```python
from build123d import *

# Parameters (mm, degrees)
BOSS_EXTRUDE1_DEPTH = 10
SKETCH3_R           = 2.25
SKETCH3_R_2         = 3
CUT_EXTRUDE1_DEPTH  = 10
SKETCH5_R           = 4
CUT_EXTRUDE2_DEPTH  = 5


with BuildPart() as part:
    # Sketch2 → Boss-Extrude1 (new body)
    with BuildSketch(Plane(origin=(0, 0, 0), x_dir=(1, 0, 0), z_dir=(0, 1, 0))):
        Polygon((0, -34), (34, 0), (94, 0), (94, -94), (0, -94), align=None)
    extrude(amount=BOSS_EXTRUDE1_DEPTH)

    # Sketch3 → Cut-Extrude1 (cut)
    with BuildSketch(Plane(origin=(0, 10, 0), x_dir=(1, 0, 0), z_dir=(0, 1, 0))):
        with Locations((58.75, -6.25)):
            Circle(SKETCH3_R)
        with Locations((87.75, -35.25)):
            Circle(SKETCH3_R)
        with Locations((6.25, -62.75)):
            Circle(SKETCH3_R)
        with Locations((31.25, -87.75)):
            Circle(SKETCH3_R)
        with Locations((6, -88)):
            Circle(SKETCH3_R_2)
        with BuildLine():
            Line((90.828427125, -7.414213562), (89.414213562, -8.828427125))
            ThreePointArc((89.414213562, -8.828427125), (85.171572875, -8.828427125), (85.171572875, -4.585786438))
            Line((85.171572875, -4.585786438), (86.585786438, -3.171572875))
            ThreePointArc((86.585786438, -3.171572875), (90.828427125, -3.171572875), (90.828427125, -7.414213562))
        make_face()
    extrude(amount=-CUT_EXTRUDE1_DEPTH, mode=Mode.SUBTRACT)

    # Sketch5 → Cut-Extrude2 (cut)
    with BuildSketch(Plane(origin=(0, 10, 0), x_dir=(1, 0, 0), z_dir=(0, 1, 0))):
        with Locations((58.75, -6.25)):
            Circle(SKETCH5_R)
        with Locations((87.75, -35.25)):
            Circle(SKETCH5_R)
        with Locations((6.25, -62.75)):
            Circle(SKETCH5_R)
        with Locations((31.25, -87.75)):
            Circle(SKETCH5_R)
    extrude(amount=-CUT_EXTRUDE2_DEPTH, mode=Mode.SUBTRACT)


solid = part.part
```
Model file for the job. Use its own axes, mm. A direction names the side the tool comes from. Coordinates: 2 decimals unless noted, no trailing zeros. Order: outer loops, then holes, each group sorted by start corner. A loop starts at its lowest first (then second) coordinate and runs counter-clockwise, first axis right, second up. Notation, with made-up numbers: (48, -5.5) -> (87, -5.5) arc R26 cw to (87, 10.5) -> close; hole circle Ø5 at (-28.75, -10.75). An arc over 180 degrees is marked (long way). Answer as a JSON object with one key per item and string values. Group by question number.
1) Flat gauge pins, fed straight in: pin 1 (4 mm diameter, centred on x = 60, z = 6.5, fed in from +Y); pin 2 (3.5 mm diameter, centred on x = 6.25, z = 62.75, fed in from +Y). Where does each tip first touch, or does it go through?
2) Cut at D-D, the plane z = 6.25. Write the cut outline in (x, y), then the cut area to 3 significant figures.
3) Cut at C-C, the plane z = 62.75. Write the cut outline in (x, y).
4) Cut at B-B, the plane x = 6. Write the cut outline in (y, z), then the cut area to 3 significant figures.
5) Drill centre lines: L1, parallel to Z at x = 6.25, y = 6.05; L2, parallel to X at y = 1.75, z = 89; L3, parallel to X at y = 2.65, z = 35.25. Where is each one in solid material? Low to high.
6) Pull direction X, two halves, no side cores. Call faces 3 (the face through (48, 5, 94)), 4 (the face through (94, 5, 46)), 5 (the face through (5.762, 2.535, 64.946)): +X half, -X half, draft (parallel to the pull), parting line (faces both ways), or undercut.
7) Cut at A-A, the plane y = 8. Write the cut outline in (x, z).
8) Which spindle directions (+Z, -Z, +X, -X, +Y, -Y) get a long thin tool onto all of the face, cutting with end or side? Do faces 1 (the face through (48, 0, 46)), 2 (the face through (30.383, 7.535, 91.655)). Say none if no direction does.
Check values:
{
 "1": {"pin 1": "stops at y = 5", "pin 2": "passes through"},
 "2": {"outline": "(27.75, 0) -> (56.5, 0) -> (56.5, 5) -> (54.75, 5) -> (54.75, 10) -> (27.75, 10) -> close; (61, 0) -> (84.33, 0) -> (84.33, 10) -> (62.75, 10) -> (62.75, 5) -> (61, 5) -> close; (91.55, 0) -> (94, 0) -> (94, 10) -> (91.55, 10) -> close", "area": "528 mm²"},
 "3": {"outline": "(0, 0) -> (4, 0) -> (4, 5) -> (2.25, 5) -> (2.25, 10) -> (0, 10) -> close; (8.5, 0) -> (94, 0) -> (94, 10) -> (10.25, 10) -> (10.25, 5) -> (8.5, 5) -> close"},
 "4": {"outline": "(0, 28) -> (10, 28) -> (10, 58.76) -> (5, 58.76) -> (5, 60.51) -> (0, 60.51) -> close; (0, 64.99) -> (5, 64.99) -> (5, 66.74) -> (10, 66.74) -> (10, 85) -> (0, 85) -> close; (0, 91) -> (10, 91) -> (10, 94) -> (0, 94) -> close", "area": "538 mm²"},
 "5": {"L1": "z = 27.75 to 58.75, 66.75 to 85.01, 90.99 to 94", "L2": "x = 0 to 3.17, 8.83 to 29.38, 33.12 to 94", "L3": "x = 0 to 85.5, 90 to 94"},
 "6": {"face 3": "draft", "face 4": "+X half", "face 5": "undercut"},
 "7": {"outline": "(0, 34) -> (34, 0) -> (94, 0) -> (94, 94) -> (0, 94) -> close; hole circle Ø8 at (6.25, 62.75); hole circle Ø6 at (6, 88); hole circle Ø8 at (31.25, 87.75); hole circle Ø8 at (58.75, 6.25); hole circle Ø8 at (87.75, 35.25); hole (85.17, 4.59) -> (86.59, 3.17) arc R3 ccw to (90.83, 7.41) -> (89.41, 8.83) arc R3 ccw to start"},
 "8": {"face 1": "+Z, -Z, +X, -X, -Y", "face 2": "+Y"}
}
